The listing builds one solid part. Answer for the finished solid, in the listing's coordinates (mm). Face numbers are marked on the shaded views. A direction names the side the tool comes from. Coordinates: 2 decimals unless noted, no trailing zeros. Write each loop counter-clockwise with the first axis right and the second up, starting at its lowest first coordinate (ties: lowest second). Pieces come first, ordered by that corner, then holes. Notation, with made-up numbers: M 78.25,-23.5 L 116.25,-23.5 A31 ccw 116.25,5.5 Z; hole C 66,-31 d7. An arc over 180 degrees is marked long. Write item = value, one per line. Start each with the question number.
```python
from build123d import *

# Parameters (mm, degrees)
SKETCH1_R           = 4.5
BOSS_EXTRUDE3_DEPTH = 4.5
CUT_EXTRUDE2_DEPTH  = 2
SKETCH5_R           = 2.5
BOSS_EXTRUDE4_DEPTH = 5


with BuildPart() as part:
    # Sketch1 → Boss-Extrude3 (new body)
    with BuildSketch(Plane.XY):
        Circle(SKETCH1_R)
    extrude(amount=BOSS_EXTRUDE3_DEPTH)

    # Sketch4 → Cut-Extrude2 (cut)
    with BuildSketch(Plane(origin=(0, 0, 0), x_dir=(-1, 0, 0), z_dir=(0, 0, -1))):
        Polygon((3.150328976, 0.094133336), (1.493642628, 2.775331592), (-1.656686348, 2.681198256), (-3.150328976, -0.094133336), (-1.493642628, -2.775331592), (1.656686348, -2.681198256), align=None)
    extrude(amount=-CUT_EXTRUDE2_DEPTH, mode=Mode.SUBTRACT)

    # Sketch5 → Boss-Extrude4 (add)
    with BuildSketch(Plane.XY.offset(4.5)):
        Circle(SKETCH5_R)
    extrude(amount=BOSS_EXTRUDE4_DEPTH)


solid = part.part
```
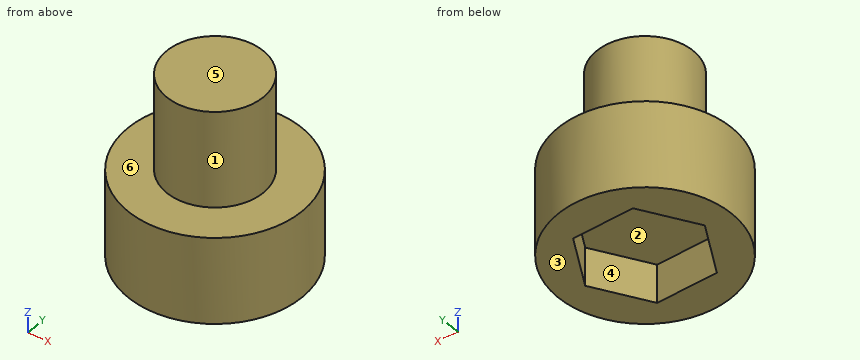
1. The part is cut by section C-C, the plane y = 0.75. Write down the section's boundary in (x, z).
2. The part is cut by section D-D, the plane z = 7.75. Write down the section's boundary in (x, y), and give its area (3 significant figures).
3. Each of these flat-tipped pins is pushed along its axis until it touches: pin 1 (1.7 mm diameter, centred on x = 1.5, y = 0.5, fed in from -Z); pin 2 (5 mm diameter, centred on x = 1.5, z = 7.5, fed in from +Y); pin 3 (4 mm diameter, centred on y = 2.5, z = 5.5, fed in from -X). Where does it stop, or does it pass through?
4. For a pull along X with two mould halves and no side action, classify the marked faces 1, 2 and 3 as pulls with the +X half, pulls with the -X half, needs draft (parallel to the pull), parting line crosses it, or undercut.
5. For the marked faces 4, 5 and 6, determine the directions among +Z, -Z, +X, -X, +Y, -Y from which every point of the face is accessible in a straight line to the end or side of a thin tool.
6. The part is cut by section A-A, the plane z = 1.25. Write down the section's boundary in (x, y), and give its area (3 significant figures).
7. Straight lines are drawn through the part: L1, parallel to Z at x = -1, y = 0.75; L2, parallel to Z at x = 1.25, y = 4.25; L3, parallel to X at y = 2.5, z = 1.5. For each, find the intervals that lie inside material, in ascending order. Write a range as [from, to].
8. The part is cut by section B-B, the plane x = -2.75. Write down the section's boundary in (y, z), and give its area (3 significant figures).
Solution:
q1.outline = M -4.44,0 L -2.75,0 L -2.75,2 L 2.7,2 L 2.7,0 L 4.44,0 L 4.44,4.5 L 2.38,4.5 L 2.38,9.5 L -2.38,9.5 L -2.38,4.5 L -4.44,4.5 Z
q2.outline = C 0,0 d5
q2.area = 19.6 mm^2
q3.pin_1 = 2
q3.pin_2 = 2.5
q3.pin_3 = -4.43
q4.face_1 = parting line crosses it
q4.face_2 = undercut
q4.face_3 = needs draft
q5.face_4 = -Z
q5.face_5 = +Z, +X, -X, +Y, -Y
q5.face_6 = +Z
q6.outline = C 0,0 d9; hole M -3.15,0.09 L -1.66,-2.68 L 1.49,-2.78 L 3.15,-0.09 L 1.66,2.68 L -1.49,2.78 Z
q6.area = 37.8 mm^2
q7.L1 = [2, 9.5]
q7.L2 = [0, 4.5]
q7.L3 = [-3.74, -1.66], [1.75, 3.74]
q8.outline = M -3.56,0 L -0.65,0 L -0.65,2 L 0.74,2 L 0.74,0 L 3.56,0 L 3.56,4.5 L -3.56,4.5 Z
q8.area = 29.3 mm^2
